Solid Edge part; units mm, degrees
sketch "Sketch1" plane through (0, 0, 0) normal (0, 0, 1) x (1, 0, 0)
  line L0 (183, -182) -> (0, -182)
  line L1 (0, -182) -> (0, 0)
  line L2 (0, 0) -> (183, 0)
  line L3 (183, 0) -> (183, -182)
extrude "Protrusion1" add sketch "Sketch1" along normal blind 20
sketch "Sketch2" plane through (91.5, -182, 10) normal (0, -1, 0) x (1, 0, 0)
  circle A0 centre (-59.5, -10) radius 16
  circle A1 centre (65.5, -10) radius 16
extrude "Cutout1" cut sketch "Sketch2" against normal through all
hole "Hole1" at (10, -172, 20) direction (0, 0, -1) diameter 10 end up to next
hole "Hole2" at (90, -172, 20) direction (0, 0, -1) diameter 10 end up to next
hole "Hole3" at (90, -10, 20) direction (0, 0, -1) diameter 10 end up to next
hole "Hole4" at (10, -10, 20) direction (0, 0, -1) diameter 10 end up to next
Model file for the job. Use its own axes, mm. Coordinates: 2 decimals unless noted, no trailing zeros. Order: outer loops, then holes, each group sorted by start corner. A loop starts at its lowest first (then second) coordinate and runs counter-clockwise, first axis right, second up. Notation, with made-up numbers: (81.5, 80.5) - (103.5, 80.5) arc R11 cw to (103.5, 85.5) - close; hole circle Ø7 at (34, 65). An arc over 180 degrees is marked (long way). Return JSON: item names as keys, results as strings. Group by question number.
1) Saw through at B-B, the plane x = 90. Write the cut outline in (y, z), plus the area to 3 significant figures.
2) Mould opens along X. For faces 1 (the cylindrical face through (85.12, -8.92, 10.14)), 2 (the flat face through (183, -90, 10)), 3 (the flat face through (95, -90, 0)) say: released by +X, released by -X, zero draft, split by the parting line, or undercut.
3) Saw through at A-A, the plane z = 12.5. Write the cut outline in (x, y), plus the area to 3 significant figures.
4) Saw through at D-D, the plane y = -100.5. Write the cut outline in (x, z), plus the area to 3 significant figures.
5) Saw through at C-C, the plane y = -172. Write the cut outline in (x, z).
6) Probe line 1 (Y direction, x = 10, z = 15.75); line 2 (X direction, y = -130, z = 3.25); line 3 (X direction, y = -30.5, z = 11). List the from-to ranges inside material, lowest first. Write a range as from..to.
Values found:
{
 "1": {"outline": "(-182, 0) - (-177, 0) - (-177, 20) - (-182, 20) - close; (-167, 0) - (-15, 0) - (-15, 20) - (-167, 20) - close; (-5, 0) - (0, 0) - (0, 20) - (-5, 20) - close", "area": "3,240 mm²"},
 "2": {"face 1": "undercut", "face 2": "released by +X", "face 3": "zero draft"},
 "3": {"outline": "(0, -182) - (22.01, -182) - (22.01, 0) - (0, 0) - close; (41.99, -182) - (147.01, -182) - (147.01, 0) - (41.99, 0) - close; (166.99, -182) - (183, -182) - (183, 0) - (166.99, 0) - close; hole circle Ø10 at (10, -172); hole circle Ø10 at (10, -10); hole circle Ø10 at (90, -172); hole circle Ø10 at (90, -10)", "area": "25,700 mm²"},
 "4": {"outline": "(0, 0) - (16, 0) arc R16 cw to (48, 0) - (141, 0) arc R16 cw to (173, 0) - (183, 0) - (183, 20) - (0, 20) - close", "area": "2,860 mm²"},
 "5": {"outline": "(0, 0) - (5, 0) - (5, 20) - (0, 20) - close; (15, 0) - (16, 0) arc R16 cw to (48, 0) - (85, 0) - (85, 20) - (15, 20) - close; (95, 0) - (141, 0) arc R16 cw to (173, 0) - (183, 0) - (183, 20) - (95, 20) - close"},
 "6": {"line 1": "y = -182..-177, -167..-15, -5..0", "line 2": "x = 0..16.33, 47.67..141.33, 172.67..183", "line 3": "x = 0..20.38, 43.62..145.38, 168.62..183"}
}
